Geometry: final body of the model. Coordinates: model frame, mm. Coordinates: 2 decimals unless noted, no trailing zeros. Loops run counter-clockwise (first coordinate to the right, second up) from the corner with the lowest first, then second, coordinate; pieces in that order, holes last. Notation, with made-up numbers: (71, 69) -> (97, 69) arc R24 ccw to (97, 90) -> close; hole circle Ø10 at (69.5, 61). An arc over 180 degrees is marked (long way). One line per item, written item: value. Start each with the question number.
Item 1: Section query D-D on x = 201.6. Return loops of the section in (y, z), then the cut area to 3 significant figures.
Item 2: Section query A-A on y = 15. Return loops of the section in (x, z).
Item 3: Section query B-B on x = 20. Return loops of the section in (y, z).
Item 4: Ray query, probe 1 along Y at (x, z) = (20, 5); probe 2 along X at (y, z) = (16.75, 9); probe 3 along X at (y, z) = (15.5, 4.5). Return the intervals inside material, ascending. Write a range as from..to.
Item 5: Section query C-C on z = 7.5. Return loops of the section in (x, y).
Item 6: Contact query for a flat-ended pin moving along its axis: pin 1 Ø2 at (x, y) = (23, 12.5) entering from +Z. Output: stop coordinate, or through.
Autodesk Inventor part; units mm, degrees
ref_plane "YZ Plane" through (0, 0, 0) normal (1, 0, 0) x (0, 1, 0)
ref_plane "XZ Plane" through (0, 0, 0) normal (0, 1, 0) x (-1, 0, 0)
ref_plane "XY Plane" through (0, 0, 0) normal (0, 0, 1) x (1, 0, 0)
sketch "Sketch1" plane through (0, 0, 0) normal (0, 0, 1) x (1, 0, 0)
  line L0 (0, 0) -> (221.6, 0)
  line L1 (221.6, 0) -> (221.6, 30)
  line L2 (221.6, 30) -> (0, 30)
  line L3 (0, 30) -> (0, 0)
  dimension "d0" = 221.6
  dimension "d1" = 30
extrude "Extrusion1" add sketch "Sketch1" along normal blind 12
fillet "Fillet1" radius 5 4 edges at (0, 30, 6) (0, 0, 6) (221.6, 0, 6) (221.6, 30, 6)
sketch "Sketch2" plane through (0, 0, 12) normal (0, 0, 1) x (1, 0, 0)
  line L0 (0, 25) -> (0, 5)
  line L1 (0, 15) -> (20, 15)
  circle A0 centre (20, 15) radius 6
  line L2 (5, 0) -> (216.6, 0)
  line L3 (110.8, 0) -> (110.8, 30)
  line L4 (216.6, 30) -> (5, 30)
  line L5 (221.6, 5) -> (221.6, 25)
  line L6 (221.6, 15) -> (201.6, 15)
  circle A1 centre (201.6, 15) radius 3
  point P0 (0, 0)
  dimension "d5" = 20
  dimension "d6" = 12
  dimension "d9" = 20
  dimension "d10" = 6
extrude "Extrusion2" cut sketch "Sketch2" against normal through all
ref_plane "Work Plane1" through (0, 0, 6) normal (0, 0, 1) x (1, 0, 0)
properties part number "Fourbar-Rocker"
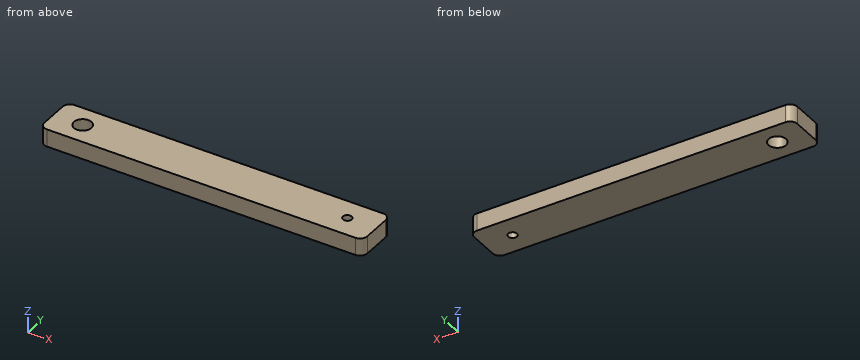
Reply:
1. outline: (0, 0) -> (12, 0) -> (12, 12) -> (0, 12) -> close; (18, 0) -> (30, 0) -> (30, 12) -> (18, 12) -> close
1. area: 288 mm²
2. outline: (0, 0) -> (14, 0) -> (14, 12) -> (0, 12) -> close; (26, 0) -> (198.6, 0) -> (198.6, 12) -> (26, 12) -> close; (204.6, 0) -> (221.6, 0) -> (221.6, 12) -> (204.6, 12) -> close
3. outline: (0, 0) -> (9, 0) -> (9, 12) -> (0, 12) -> close; (21, 0) -> (30, 0) -> (30, 12) -> (21, 12) -> close
4. probe 1: y = 0..9, 21..30
4. probe 2: x = 0..14.26, 25.74..199.16, 204.04..221.6
4. probe 3: x = 0..14.02, 25.98..198.64, 204.56..221.6
5. outline: (0, 5) arc R5 ccw to (5, 0) -> (216.6, 0) arc R5 ccw to (221.6, 5) -> (221.6, 25) arc R5 ccw to (216.6, 30) -> (5, 30) arc R5 ccw to (0, 25) -> close; hole circle Ø12 at (20, 15); hole circle Ø6 at (201.6, 15)
6. pin 1: passes through
